Design review of the part built by this model. Coordinates are the model's own, in mm. Face numbers are marked on the shaded views. A direction names the side the tool comes from. Round coordinates to 2 decimals unless told otherwise and drop trailing zeros. Order: outer loops, then holes, each group sorted by start corner. A loop starts at its lowest first (then second) coordinate and runs counter-clockwise, first axis right, second up. Notation, with made-up numbers: M 63,5.5 L 114,5.5 A22 ccw 114,27.5 Z; hole C 41.5,8 d5. An arc over 180 degrees is marked long. Use a Markdown table: item, result. Add a question column.
(1) Machinability: for the marked faces 1 and 2, which of the approach directions +Z, -Z, +X, -X, +Y, -Y give a long, thin tool a straight path to every point of the face, cutting with its end or side? Answer none if there is none.
(2) Take a section at D-D (y = 192). Write out the cut boundary in (x, z), then the cut area to 3 significant figures.
(3) To check wall thickness, follow probe 1 along X at (y, z) = (203.2, 8.75) (3 decimals); probe 2 along Y at (x, z) = (4, 2); probe 3 along X at (y, z) = (6, 12). State the ranges of each line that lie inside material, in increasing order. Write a range as from..to.
(4) Take a section at A-A (z = 6.35). Count the separate pieces of the cut face and the enclosed holes in it, then the cut area to 3 significant figures.
(5) Take a section at C-C (y = 73). Write out the cut boundary in (x, z).
(6) The part is to be moulded in two halves that separate along X. For the marked faces 3, 4 and 5, say which applies: released by +X, released by -X, zero draft, split by the parting line, or undercut.
(7) For pin 1 (5 mm diameter, centred on y = -17.5, z = 5.5, fed in from -X); pin 2 (6 mm diameter, centred on y = 146.5, z = 8.5, fed in from +X); pin 3 (4 mm diameter, centred on x = 14, z = 10.5, fed in from -Y); pin 4 (5 mm diameter, centred on x = 0, y = 203.2, fed in from -Z), all flat-tipped, find the tip position at first contact; note any pin that passes through.
```python
from build123d import *

# Parameters (mm, degrees)
F0_R          = 3.175
F1_DEPTH      = 12.7
F2_R          = 3.175
F3_DEPTH      = 25.4
F4_R          = 2.38125
F5_DEPTH      = 6.35
F5_DEPTH_BACK = 22.8610001193
F7_R          = 4.7625
F8_DEPTH      = 10.16


with BuildPart() as f1:
    # F0 (on Top) → F1 (new body)
    with BuildSketch(Plane.XY):
        with BuildLine():
            Line((-9.5044674936, 203.825078125), (-22.8107219847, 1.5001875))
            ThreePointArc((-22.8107219847, 1.5001875), (-17.219220581, -15.035891812), (-1.5875, -22.8048118552))
            Line((-1.5875, -22.8048118552), (-1.5875, -12.6003906189))
            ThreePointArc((-1.5875, -12.6003906189), (-6.3798128297, -10.981256224), (-10.16, -7.62))
            Line((-10.16, -7.62), (-10.16, 7.62))
            ThreePointArc((-10.16, 7.62), (0, 12.7), (10.16, 7.62))
            Line((10.16, 7.62), (10.16, -7.62))
            ThreePointArc((10.16, -7.62), (6.3798128297, -10.981256224), (1.5875, -12.6003906189))
            Line((1.5875, -12.6003906189), (1.5875, -22.8048118552))
            ThreePointArc((1.5875, -22.8048118552), (17.219220581, -15.035891812), (22.8107219847, 1.5001875))
            Line((22.8107219847, 1.5001875), (9.5044674936, 203.825078125))
            ThreePointArc((9.5044674936, 203.825078125), (0, 212.725), (-9.5044674936, 203.825078125))
        make_face()
        with BuildLine():
            ThreePointArc((9.3460597021, 51.4146601563), (0, 41.43375), (-9.3460597021, 51.4146601563))
            Line((-9.3460597021, 51.4146601563), (-4.3562142679, 127.2864941406))
            ThreePointArc((-4.3562142679, 127.2864941406), (0, 131.365625), (4.3562142679, 127.2864941406))
            Line((4.3562142679, 127.2864941406), (9.3460597021, 51.4146601563))
        make_face(mode=Mode.SUBTRACT)
        with Locations((0, 203.2)):
            Circle(F0_R, mode=Mode.SUBTRACT)
    extrude(amount=F1_DEPTH)

    # F2 (on face) → F3 (cut)
    with BuildSketch(Plane.YZ.offset(-10.16)):
        with Locations((0, 6.35)):
            Circle(F2_R)
    extrude(amount=-F3_DEPTH, mode=Mode.SUBTRACT)

    # F4 (on Right) → F5 (cut, two sides)
    with BuildSketch(Plane.YZ) as f5_sk:
        with Locations((-17.7026012371, 6.35)):
            Circle(F4_R)
    extrude(amount=F5_DEPTH, mode=Mode.SUBTRACT)
    extrude(f5_sk.sketch, amount=-F5_DEPTH_BACK, mode=Mode.SUBTRACT)

    # F7 (on offset) → F8 (cut)
    with BuildSketch(Plane.YZ.offset(-20.6375)):
        with Locations((-17.7026012371, 6.35)):
            Circle(F7_R)
    extrude(amount=F8_DEPTH, mode=Mode.SUBTRACT)


solid = f1.part
```
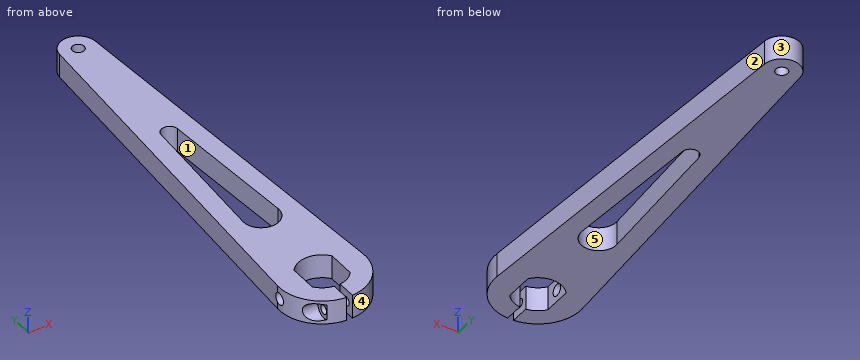
Verdict:
| question | item | result |
|---|---|---|
| 1 | face 1 | +Z, -Z |
| 1 | face 2 | +Z, -Z, +X, +Y |
| 2 | outline | M -10.28,0 L 10.28,0 L 10.28,12.7 L -10.28,12.7 Z |
| 2 | area | 261 mm^2 |
| 3 | probe 1 | x = -9.546..-3.175, 3.175..9.546 |
| 3 | probe 2 | y = -22.51..-12.05, 12.05..42.33, 128.75..211.84 |
| 3 | probe 3 | x = -22.51..-10.16, 10.16..22.51 |
| 4 | separate pieces | 3 |
| 4 | enclosed holes | 2 |
| 4 | area | 5,640 mm^2 |
| 5 | outline | M -18.11,0 L -7.93,0 L -7.93,12.7 L -18.11,12.7 Z; M 7.93,0 L 18.11,0 L 18.11,12.7 L 7.93,12.7 Z |
| 6 | face 3 | split by the parting line |
| 6 | face 4 | released by +X |
| 6 | face 5 | undercut |
| 7 | pin 1 | stops at x = -10.48 |
| 7 | pin 2 | stops at x = 13.47 |
| 7 | pin 3 | stops at y = -19.46 |
| 7 | pin 4 | passes through |
